from build123d import *

# Parameters (mm, degrees)
SKETCH_R  = 15
PAD_DEPTH = 3


with BuildPart() as part:
    # Sketch → Pad (new body)
    with BuildSketch(Plane.XY):
        Polygon((-15.146858, 7.474872), (-16.445896, 8.224872), (-15.345896, 10.130128), (-14.046858, 9.380128), (-12.696102, 11.140467), (-13.756762, 12.201128), (-12.201128, 13.756762), (-11.140467, 12.696102), (-9.380128, 14.046858), (-10.130128, 15.345896), (-8.224872, 16.445896), (-7.474872, 15.146858), (-5.424913, 15.995979), (-5.813142, 17.444868), (-3.688105, 18.014269), (-3.299877, 16.565381), (-1.1, 16.855), (-1.1, 18.355), (1.1, 18.355), (1.1, 16.855), (3.299877, 16.565381), (3.688105, 18.014269), (5.813142, 17.444868), (5.424913, 15.995979), (7.474872, 15.146858), (8.224872, 16.445896), (10.130128, 15.345896), (9.380128, 14.046858), (11.140467, 12.696102), (12.201128, 13.756762), (13.756762, 12.201128), (12.696102, 11.140467), (14.046858, 9.380128), (15.345896, 10.130128), (16.445896, 8.224872), (15.146858, 7.474872), (15.997323, 5.424913), (17.446213, 5.813142), (18.015614, 3.688105), (16.566725, 3.299877), (16.854909, 1.1), (18.35491, 1.1), (18.355, -1.1), (16.85491, -1.1), (16.566725, -3.299877), (18.015614, -3.688105), (17.446212, -5.813142), (15.997323, -5.424913), (15.146858, -7.474872), (16.445896, -8.224872), (15.345896, -10.130128), (14.046858, -9.380128), (12.696102, -11.140467), (13.756762, -12.201128), (12.201128, -13.756762), (11.140467, -12.696102), (9.380128, -14.046858), (10.130128, -15.345896), (8.224872, -16.445896), (7.474872, -15.146858), (5.424913, -15.995979), (5.813142, -17.444868), (3.688105, -18.014269), (3.299877, -16.565381), (1.1, -16.855), (1.1, -18.355), (-1.1, -18.355), (-1.1, -16.855), (-3.299877, -16.565381), (-3.688105, -18.014269), (-5.813142, -17.444868), (-5.424913, -15.995979), (-7.474872, -15.146858), (-8.224872, -16.445896), (-10.130128, -15.345896), (-9.380128, -14.046858), (-11.140467, -12.696102), (-12.201128, -13.756762), (-13.756762, -12.201128), (-12.696102, -11.140467), (-14.046858, -9.380128), (-15.345896, -10.130128), (-16.445896, -8.224872), (-15.146858, -7.474872), (-15.997323, -5.424913), (-17.446212, -5.813142), (-18.015614, -3.688105), (-16.566725, -3.299877), (-16.854909, -1.1), (-18.354909, -1.1), (-18.354909, 1.1), (-16.854909, 1.1), (-16.566725, 3.299877), (-18.015614, 3.688105), (-17.446212, 5.813142), (-15.997323, 5.424913), align=None)
        Circle(SKETCH_R, mode=Mode.SUBTRACT)
    extrude(amount=PAD_DEPTH)


solid = part.part
Can you work these out from the model? Positions are in its coordinate system, mm. A direction names the side the tool comes from. Round coordinates to 2 decimals unless told otherwise and drop trailing zeros. Write each loop counter-clockwise with the first axis right and the second up, starting at its lowest first coordinate (ties: lowest second). Pieces come first, ordered by that corner, then holes. Notation, with made-up numbers: (2, 25.25) -> (54, 25.25) arc R33 ccw to (54, 63.25) -> close; hole circle Ø6 at (-22.75, 19.25). An arc over 180 degrees is marked (long way). Use one line per item in the form item = value. Start each with the question number.
Q1. Imagine slicing it at B-B (y = 6.5). Please give me the cut outline in (x, z), then the cut area to 3 significant figures.
Q2. Imagine slicing it at A-A (x = 0). Please give me the cut outline in (y, z) (3 decimals), then the cut area to 3 significant figures.
Q3. Which directions (+Z, -Z, +X, -X, +Y, -Y) give clear straight access to the entire face, cutting with the end or side of a thin tool? Please do faces 4 (the face through (-14.705, 9.76, 1.479)), 5 (the face through (13.219, -11.663, 1.479)), 6 (the face through (-13.219, 11.663, 1.479)).
Q4. I'm going to push flat-ended pins straight in: P1, Ø0.8, axis at x = 17.5, z = 2, coming from the +Y side; P2, Ø4, axis at x = 1, y = -11, coming from the -Z side; P3, Ø1.2, axis at y = 17.5, z = 1, coming from the +X side; P4, Ø1.7, axis at x = 17.5, z = 2, coming from the -Y side. Where does each tip first touch, or does it pass through?
Q5. If I drill on probe 1 along Y at (x, z) = (0, 0.75) (3 decimals); probe 2 along X at (y, z) = (-13, 2.65); probe 3 along Y at (x, z) = (15.5, 1.9), over which ranges is the centre line in solid material (lowest first)? Write a range as [from, to].
Q6. We'd pull the mould along X, two halves only. Please class faces 1 (the face through (16, 9, 1)), 2 (the face through (15.57, 6.46, 1.48)), 3 (the face through (15, 3, 0)): +X half, -X half, draft (parallel to the pull), parting line (faces both ways), or undercut.
Worked out:
q1.outline = (-15.55, 0) -> (-13.52, 0) -> (-13.52, 3) -> (-15.55, 3) -> close; (13.52, 0) -> (15.55, 0) -> (15.55, 3) -> (13.52, 3) -> close
q1.area = 12.2 mm^2
q2.outline = (-18.355, 0) -> (-15, 0) -> (-15, 3) -> (-18.355, 3) -> close; (15, 0) -> (18.355, 0) -> (18.355, 3) -> (15, 3) -> close
q2.area = 20.1 mm^2
q3.face_4 = +Z, -Z, +Y
q3.face_5 = +Z, -Z, +X
q3.face_6 = +Z, -Z, -X
q4.P1 = 5.81
q4.P2 = through
q4.P3 = 5.81
q4.P4 = -5.81
q5.probe_1 = [-18.355, -15], [15, 18.355]
q5.probe_2 = [-12.96, -11.44], [-10.74, -7.48], [7.48, 10.74], [11.44, 12.96]
q5.probe_3 = [-9.86, -7.68], [-6.62, 6.62], [7.68, 9.86]
q6.face_1 = +X half
q6.face_2 = undercut
q6.face_3 = draft
